Check sheet for the drawn part. Datum: minimum x, y, z corner. Units: mm. Round coordinates to 2 decimals unless told otherwise and drop trailing zeros. Order: outer loops, then holes, each group sorted by start corner. A loop starts at its lowest first (then second) coordinate and runs counter-clockwise, first axis right, second up. Notation, with made-up numbers: (-33, 79.25) -> (7, 79.25) arc R13 ccw to (7, 92.25) -> close; hole circle Ø5 at (26.5, 0.5). An arc over 180 degrees is marked (long way). Answer in a Markdown table with one row per item.
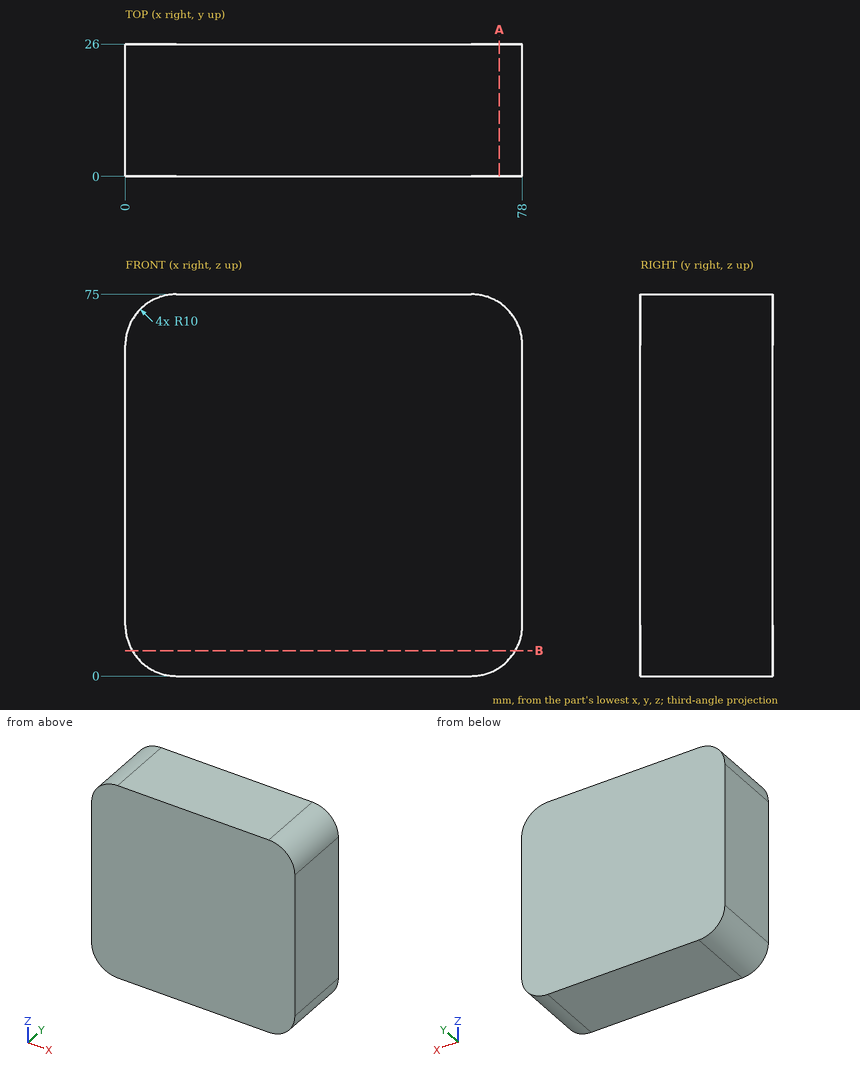
(1) Depth check by flat-ended pin: pin 1 Ø5 at (x, z) = (48.5, 37) entering from -Y. Enter the tip coordinate at first touch or a pass-through.
Solutions:
| item | result |
|---|---|
| pin 1 | y = 0 |
(2) Section check B-B on z = 5. Record the boundary of the cut face in (x, y), plus the area to 3 significant figures.
Solutions:
| item | result |
|---|---|
| outline | (1.34, 0) -> (76.66, 0) -> (76.66, 26) -> (1.34, 26) -> close |
| area | 1,960 mm^2 |
(3) Scan lines: probe 1 along X at (y, z) = (10, 4); probe 2 along Z at (x, y) = (73.5, 7); probe 3 along X at (y, z) = (7.5, 4.5). Record each from-to range of solid material in increasing order. Write a range as from..to.
Solutions:
| item | result |
|---|---|
| probe 1 | 2..76 |
| probe 2 | 1.65..73.35 |
| probe 3 | 1.65..76.35 |
(4) Section check A-A on x = 73.5. Record the boundary of the cut face in (y, z).
Solutions:
| item | result |
|---|---|
| outline | (0, 1.65) -> (26, 1.65) -> (26, 73.35) -> (0, 73.35) -> close |
